Read the model definition and answer for the solid it produces. Units are mm, in the model's axes. A direction names the side the tool comes from. Give positions to 0.01 mm unless a question says otherwise; leave off trailing zeros. Order: outer loops, then holes, each group sorted by start corner. A loop starts at its lowest first (then second) coordinate and runs counter-clockwise, first axis right, second up.
```python
from build123d import *

# Parameters (mm, degrees)
SKETCH_1_R             = 65
EXTRUDE_1_DEPTH        = 5
SKETCH_2_R             = 50
EXTRUDE_2_DEPTH        = 7
SKETCH_3_R             = 1.6
CUT_EXTRUDE_1_DEPTH    = 58
SKETCH_4_R             = 12.5
CUT_EXTRUDE_2_DEPTH    = 93.703829479
SKETCH_5_R             = 45
SKETCH_5_R_2           = 40
EXTRUDE_3_DEPTH        = 13
HOLE_WIZARD_M3_1_D     = 2.5
SKETCH_9_R             = 1.6
CUT_EXTRUDE_3_DEPTH    = 10
HOLE_WIZARD_M4_3_D     = 3.3
HOLE_WIZARD_M4_3_DEPTH = 9.5
HOLE_WIZARD_M4_3_TIP   = 0.991420021


with BuildPart() as part:
    # 草图1 → 凸台-拉伸1 (new body)
    with BuildSketch(Plane(origin=(0, 0, 0), x_dir=(1, 0, 0), z_dir=(0, 1, 0))):
        with Locations(Location((0, 0, 0), (0, 0, 270))):
            Circle(SKETCH_1_R)
    extrude(amount=EXTRUDE_1_DEPTH)

    # 草图2 → 凸台-拉伸2 (add)
    with BuildSketch(Plane(origin=(0, 0, 0), x_dir=(-1, 0, 0), z_dir=(0, -1, 0))):
        with Locations(Location((0, 0, 0), (0, 0, 90))):
            Circle(SKETCH_2_R)
    extrude(amount=EXTRUDE_2_DEPTH)

    # 草图3 → 切除-拉伸1 (cut)
    with BuildSketch(Plane(origin=(0, 5, 0), x_dir=(1, 0, 0), z_dir=(0, 1, 0))):
        with Locations(Location((0, 20, 0), (0, 0, 270))):
            Circle(SKETCH_3_R)
        with Locations(Location((17.320508076, -10, 0), (0, 0, 270))):
            Circle(SKETCH_3_R)
        with Locations(Location((-17.320508076, -10, 0), (0, 0, 270))):
            Circle(SKETCH_3_R)
    extrude(amount=-CUT_EXTRUDE_1_DEPTH, mode=Mode.SUBTRACT)

    # 草图4 → 切除-拉伸2 (cut, through all)
    with BuildSketch(Plane(origin=(0, -7, 0), x_dir=(-1, 0, 0), z_dir=(0, -1, 0))):
        with Locations(Location((0, 0, 0), (0, 0, 90))):
            Circle(SKETCH_4_R)
    extrude(amount=-CUT_EXTRUDE_2_DEPTH, mode=Mode.SUBTRACT)

    # 草图5 → 凸台-拉伸3 (add)
    with BuildSketch(Plane(origin=(0, -7, 0), x_dir=(-1, 0, 0), z_dir=(0, -1, 0))):
        with Locations(Location((0, 0, 0), (0, 0, 270))):
            Circle(SKETCH_5_R)
        with Locations(Location((0, 0, 0), (0, 0, 270))):
            Circle(SKETCH_5_R_2, mode=Mode.SUBTRACT)
    extrude(amount=EXTRUDE_3_DEPTH)

    # M3 螺纹孔1 (through all)
    with Locations(Plane(origin=(0, -20, 42.5), x_dir=(0, 0, -1), z_dir=(0, -1, 0))):
        with Locations((0, 0), (42.5, -42.5), (85, 0), (42.5, 42.5)):
            Hole(HOLE_WIZARD_M3_1_D / 2)

    # 草图9 → 切除-拉伸3 (cut)
    with BuildSketch(Plane(origin=(0, 5, 0), x_dir=(1, 0, 0), z_dir=(0, 1, 0))):
        with Locations(Location((0, 52.5, 0), (0, 0, 270))):
            Circle(SKETCH_9_R)
        with Locations(Location((37.123106012, 37.123106012, 0), (0, 0, 270))):
            Circle(SKETCH_9_R)
        with Locations(Location((52.5, 0, 0), (0, 0, 270))):
            Circle(SKETCH_9_R)
        with Locations(Location((37.123106012, -37.123106012, 0), (0, 0, 270))):
            Circle(SKETCH_9_R)
        with Locations(Location((0, -52.5, 0), (0, 0, 270))):
            Circle(SKETCH_9_R)
        with Locations(Location((-37.123106012, -37.123106012, 0), (0, 0, 270))):
            Circle(SKETCH_9_R)
        with Locations(Location((-52.5, 0, 0), (0, 0, 270))):
            Circle(SKETCH_9_R)
        with Locations(Location((-37.123106012, 37.123106012, 0), (0, 0, 270))):
            Circle(SKETCH_9_R)
    extrude(amount=-CUT_EXTRUDE_3_DEPTH, mode=Mode.SUBTRACT)

    # M4 螺纹孔3
    with Locations(Plane(origin=(0, 5, -52.5), x_dir=(0, 0, 1), z_dir=(0, 1, 0))):
        with Locations((0, 0), (15.376893988, 37.123106012), (52.5, 52.5), (89.623106012, 37.123106012), (105, 0), (89.623106012, -37.123106012), (52.5, -52.5), (15.376893988, -37.123106012)):
            Hole(HOLE_WIZARD_M4_3_D / 2, depth=HOLE_WIZARD_M4_3_DEPTH)
            with Locations((0, 0, -(HOLE_WIZARD_M4_3_DEPTH + HOLE_WIZARD_M4_3_TIP / 2))):  # 118° drill point
                Cone(0, HOLE_WIZARD_M4_3_D / 2, HOLE_WIZARD_M4_3_TIP, mode=Mode.SUBTRACT)


solid = part.part
```
1) Given pin 1 (5.5 mm diameter, centred on x = 37.12, z = 37.12, fed in from -Y); pin 2 (10 mm diameter, centred on x = 33.5, y = -1, fed in from +Z); pin 3 (3 mm diameter, centred on x = -42.5, z = 0, fed in from +Y); pin 4 (2 mm diameter, centred on y = -13, z = 6.5, fed in from +X), each flat-ended and moving along its own axis, determine where each tip first touches the part or whether it passes through.
Final values:
pin 1: stops at y = -7
pin 2: stops at z = 58.37
pin 3: stops at y = 5
pin 4: stops at x = 44.66
2) Consider L1, parallel to Y at x = -52, z = -20; L2, parallel to X at y = -5, z = 10; L3, parallel to Y at x = 3, z = 19.5. Determine where each line is inside the solid, lowest interval first.
Final values:
L1: y = 0 to 5
L2: x = -48.99 to -18.92, -15.72 to -7.5, 7.5 to 15.72, 18.92 to 48.99
L3: y = -7 to 5
3) The part is cut by section A-A on y = -12.5. Determine the outline of the cut face in (x, z), and give its area (3 significant figures).
Final values:
outline: circle Ø90 at (0, 0); hole circle Ø2.5 at (-42.5, 0); hole circle Ø80 at (0, 0); hole circle Ø2.5 at (0, -42.5); hole circle Ø2.5 at (0, 42.5); hole circle Ø2.5 at (42.5, 0)
area: 1,320 mm2
4) For a pull along Z with two mould halves and no side action, classify faces 3 (the face through (-48, 0, -15)), 4 (the face through (15.02, -3.45, -47.69)), 5 (the face through (3.755, -1.084, -11.923)) as released by +Z, released by -Z, zero draft, split by the parting line, or undercut.
Final values:
face 3: zero draft
face 4: split by the parting line
face 5: undercut
5) The part is cut by section D-D on y = -2. Count the separate pieces of the cut face and the enclosed holes in it, and give its area (3 significant figures).
Final values:
separate pieces: 1
enclosed holes: 8
area: 7,320 mm2
6) A tool of negligible diameter and unlimited length cuts with its end or side. For faces 1 (the face through (1, 5, 14)), 2 (the face through (9, -7, 9)), from which of +Z, -Z, +X, -X, +Y, -Y can it reach the whole face along a straight path? Write none if from no direction.
Final values:
face 1: +Z, -Z, +X, -X, +Y
face 2: -Y
7) The part is cut by section B-B on z = -52.5. Determine the outline of the cut face in (x, y).
Final values:
outline: (-38.32, 0) - (-1.65, 0) - (-1.65, 5) - (-38.32, 5) - close; (1.65, 0) - (38.32, 0) - (38.32, 5) - (1.65, 5) - close
8) The part is cut by section C-C on x = -52.5. Determine the outline of the cut face in (y, z), and give its area (3 significant figures).
Final values:
outline: (0, -38.32) - (5, -38.32) - (5, -1.65) - (0, -1.65) - close; (0, 1.65) - (5, 1.65) - (5, 38.32) - (0, 38.32) - close
area: 367 mm2
